Can you work these out from the model? Positions are in its coordinate system, mm. Round coordinates to 2 decimals unless told otherwise and drop trailing zeros. Loops run counter-clockwise (first coordinate to the right, second up) from the corner with the lowest first, then second, coordinate; pieces in that order, holes last. Notation, with made-up numbers: M 65,-3 L 88,-3 A16 cw 88,17 Z; hole C 36.25,5 d1. An arc over 180 degrees is marked long. Answer as CSV lines item,"result".
from build123d import *

# Parameters (mm, degrees)
SKETCH1_W               = 15
SKETCH1_H               = 5
BOSS_EXTRUDE1_DEPTH     = 4
CUT_EXTRUDE1_DEPTH      = 13.172355436
CUT_EXTRUDE1_DEPTH_BACK = 13.172355436
SKETCH2_R               = 1.5
SKETCH3_R               = 1.55
CUT_EXTRUDE2_DEPTH      = 12.4586554
FILLET1_R               = 1


with BuildPart() as part:
    # Sketch1 → Boss-Extrude1 (new body)
    with BuildSketch(Plane(origin=(0, 0, 0), x_dir=(1, 0, 0), z_dir=(0, 1, 0))):
        with Locations((2.852112676, 0.352112676)):
            Rectangle(SKETCH1_W, SKETCH1_H)
    extrude(amount=BOSS_EXTRUDE1_DEPTH)

    # Sketch2 → Cut-Extrude1 (cut, two sides: drawn at the far end of the back side and taken through both)
    with BuildSketch(Plane(origin=(0, 0, -2.852112676), x_dir=(-1, 0, 0), z_dir=(0, 0, -1)).offset(-CUT_EXTRUDE1_DEPTH_BACK)):
        with Locations((-2.852112676, 4)):
            Circle(SKETCH2_R)
    extrude(amount=CUT_EXTRUDE1_DEPTH + CUT_EXTRUDE1_DEPTH_BACK, mode=Mode.SUBTRACT)

    # Sketch3 → Cut-Extrude2 (cut, through all)
    with BuildSketch(Plane(origin=(0, 4, 0), x_dir=(1, 0, 0), z_dir=(0, 1, 0))):
        with Locations(Location((-1.647887324, 0.352112676, 0), (0, 0, 270))):
            Circle(SKETCH3_R)
        with Locations(Location((7.352112676, 0.352112676, 0), (0, 0, 270))):
            Circle(SKETCH3_R)
    extrude(amount=-CUT_EXTRUDE2_DEPTH, mode=Mode.SUBTRACT)

    # Fillet1
    fillet1_edges = [part.edges().sort_by_distance(p)[0] for p in [
        (-4.647887324, 2, -2.852112676),
        (10.352112676, 2, -2.852112676),
        (10.352112676, 2, 2.147887324),
        (-4.647887324, 2, 2.147887324),
    ]]
    fillet(fillet1_edges, radius=FILLET1_R)


solid = part.part
Item 1: If we section it at B-B on x = -0.75: Write out the boundary of the cut face in (y, z).
Output:
outline,"M 0,-2.85 L 4,-2.85 L 4,-1.62 L 0,-1.62 Z; M 0,0.91 L 4,0.91 L 4,2.15 L 0,2.15 Z"
Item 2: We'd pull the mould along X, two halves only. Please class faces 1 (the face through (0, 4, 1)), 2 (the face through (-4.648, 2, 0)), 3 (the face through (-2.24, 2.03, 1.08)), 4 (the face through (10.05, 2.03, -2.57)): released by +X, released by -X, zero draft, split by the parting line, or undercut.
Output:
face 1,"zero draft"
face 2,"released by -X"
face 3,"undercut"
face 4,"released by +X"
Item 3: If we section it at A-A on y = 3.5: Write out the boundary of the cut face in (x, z).
Output:
outline,"M -4.65,-1.85 A1 ccw -3.65,-2.85 L 1.44,-2.85 L 1.44,2.15 L -3.65,2.15 A1 ccw -4.65,1.15 Z; M 4.27,-2.85 L 9.35,-2.85 A1 ccw 10.35,-1.85 L 10.35,1.15 A1 ccw 9.35,2.15 L 4.27,2.15 Z; hole C -1.65,-0.35 d3.1; hole C 7.35,-0.35 d3.1"
Item 4: If we section it at D-D on y = 2: Write out the boundary of the cut face in (x, z), then the cut area to 3 significant figures.
Output:
outline,"M -4.65,-1.85 A1 ccw -3.65,-2.85 L 9.35,-2.85 A1 ccw 10.35,-1.85 L 10.35,1.15 A1 ccw 9.35,2.15 L -3.65,2.15 A1 ccw -4.65,1.15 Z; hole C -1.65,-0.35 d3.1; hole C 7.35,-0.35 d3.1"
area,"59.0 mm2"
Item 5: If I drill on line 1 along X through (y, z) = (3.8, 0.3); line 2 along X through (y, z) = (0.95, -1.7); line 3 along X through (y, z) = (0.8, -0.2), over which ranges is the centre line in solid material (lowest first)? Write a range as from..to.
Output:
line 1,"x = -4.65..-3.05, -0.24..1.37, 4.34..5.95, 8.76..10.35"
line 2,"x = -4.65..-2.41, -0.88..6.59, 8.12..10.35"
line 3,"x = -4.65..-3.19, -0.11..5.81, 8.89..10.35"
Item 6: If we section it at C-C on z = 0: Write out the boundary of the cut face in (x, y), then the cut area to 3 significant figures.
Output:
outline,"M -4.65,0 L -3.16,0 L -3.16,4 L -4.65,4 Z; M -0.14,0 L 5.84,0 L 5.84,4 L 4.35,4 A1.5 cw 1.35,4 L -0.14,4 Z; M 8.86,0 L 10.35,0 L 10.35,4 L 8.86,4 Z"
area,"32.3 mm2"
